Autodesk Inventor part; units mm, degrees
ref_plane "YZ Plane" through (0, 0, 0) normal (1, 0, 0) x (0, 1, 0)
ref_plane "XZ Plane" through (0, 0, 0) normal (0, 1, 0) x (-1, 0, 0)
ref_plane "XY Plane" through (0, 0, 0) normal (0, 0, 1) x (1, 0, 0)
sketch "Sketch1" plane through (0, 0, 0) normal (0, 1, 0) x (-1, 0, 0)
  line L0 (-15, -41.5) -> (15, -41.5)
  line L1 (15, -41.5) -> (15, 41.5)
  line L2 (15, 41.5) -> (-15, 41.5)
  line L3 (-15, 41.5) -> (-15, -41.5)
  line L4 (-15, -41.5) -> (15, 41.5) construction
  line L5 (15, -41.5) -> (-15, 41.5) construction
  point P0 (0, 0)
  dimension "d0" = 30
  dimension "d1" = 83
extrude "Extrusion1" add sketch "Sketch1" along normal blind 24
sketch "Sketch2" plane through (0, 24, 0) normal (0, 1, 0) x (1, 0, 0)
  line L0 (-15, 41.5) -> (-15, -41.5)
  line L1 (-15, -41.5) -> (15, -41.5)
  point P0 (0, 0)
  point P1 (0, -32.5)
  point P2 (0, 32.5)
  dimension "d4" = 15
  dimension "d6" = 9
  dimension "d14" = 65
  dimension "d15" = 15
hole "Hole1" at (0, 24, 32.5) at (0, 24, -32.5) direction (0, -1, 0) diameter 7.134 end through all
properties part number "Pillow_support" material "Stainless Steel"
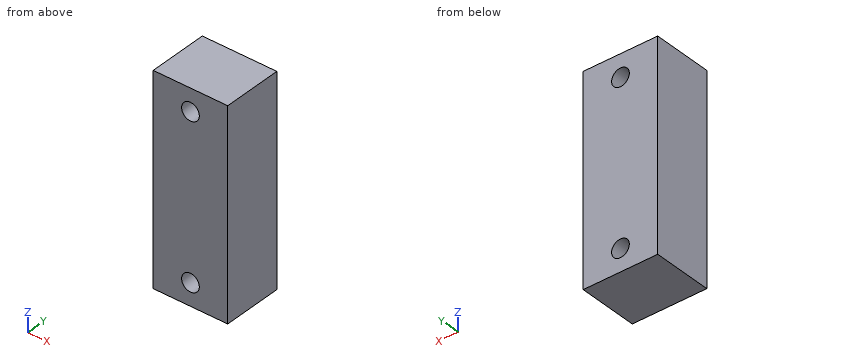
Design review of the part built by this model. Coordinates are the model's own, in mm. Give positions to 0.01 mm unless a question says otherwise; leave off trailing zeros. Write each loop counter-clockwise with the first axis right and the second up, starting at its lowest first coordinate (ties: lowest second). Pieces come first, ordered by that corner, then holes. Notation, with made-up numbers: M -33.5,27.25 L -21.5,27.25 A13 cw -21.5,49.25 Z; hole C 21,20 d8. An arc over 180 degrees is marked long. Answer as a JSON object with one key per item and string values. Group by question number.
1) We need section B-B (x = 0). Give the boundary of the cut face in (y, z), and give its area (3 significant figures).
2) For line 1 along Z through (x, y) = (0, 7.75); line 2 along X through (y, z) = (5, 32.5); line 3 along Z through (x, y) = (-1.5, 12.5), list the stretches that pass through material, from the lowest coordinate up.
3) We need section C-C (y = 19.5). Give the boundary of the cut face in (x, z).
4) We need section A-A (z = 32.5). Give the boundary of the cut face in (x, y), and give its area (3 significant figures).
5) Clearance check with a flat-ended pin moving along its axis: pin 1 Ø4.5 at (x, z) = (0, -32.5) entering from +Y. State where the tip first meets the part, or that it passes through.
Answer key:
{
 "1": {"outline": "M 0,-41.5 L 24,-41.5 L 24,-36.07 L 0,-36.07 Z; M 0,-28.93 L 24,-28.93 L 24,28.93 L 0,28.93 Z; M 0,36.07 L 24,36.07 L 24,41.5 L 0,41.5 Z", "area": "1,650 mm²"},
 "2": {"line 1": "z = -41.5 to -36.07, -28.93 to 28.93, 36.07 to 41.5", "line 2": "x = -15 to -3.57, 3.57 to 15", "line 3": "z = -41.5 to -35.74, -29.26 to 29.26, 35.74 to 41.5"},
 "3": {"outline": "M -15,-41.5 L 15,-41.5 L 15,41.5 L -15,41.5 Z; hole C 0,-32.5 d7.13; hole C 0,32.5 d7.13"},
 "4": {"outline": "M -15,0 L -3.57,0 L -3.57,24 L -15,24 Z; M 3.57,0 L 15,0 L 15,24 L 3.57,24 Z", "area": "549 mm²"},
 "5": {"pin 1": "passes through"}
}
